Design review of the part built by this model. Coordinates are the model's own, in mm. Face numbers are marked on the shaded views. A direction names the side the tool comes from. Coordinates: 2 decimals unless noted, no trailing zeros. Order: outer loops, then holes, each group sorted by start corner. A loop starts at its lowest first (then second) coordinate and runs counter-clockwise, first axis right, second up. Notation, with made-up numbers: (-34, 72.5) -> (-11, 72.5) arc R19 ccw to (-11, 80.5) -> close; hole circle Ø2 at (-28.75, 72.5). An arc over 180 degrees is marked (long way). Use a Markdown table: item, result. Add a question column.
Q1. Add section C-C (y = 17.5). State the section outline as (x, z) points (3 decimals).
Q2. Add section B-B (z = 5). State the section outline as (x, y) points (3 decimals).
Q3. Add section A-A (x = -2.5). State the section outline as (y, z) points (3 decimals), then the cut area to 3 significant figures.
Q4. The part is to be moulded in two halves that separate along X. For the marked faces 3, 4 and 5, say which applies: pulls with the +X half, pulls with the -X half, needs draft (parallel to the pull), parting line crosses it, or undercut.
Q5. Wall thickness on probe 1 along X at (y, z) = (3.25, -34.5) (3 decimals); probe 2 along X at (y, z) = (2, 7.5) (3 decimals); probe 3 along Z at (x, y) = (34, 3.25) (3 decimals): over which ranges is each line inside the solid? List them lowest first.
Q6. Machinability: for the marked faces 1 and 2, which of the approach directions +Z, -Z, +X, -X, +Y, -Y give a long, thin tool a straight path to every point of the face, cutting with its end or side? Answer none if there is none.
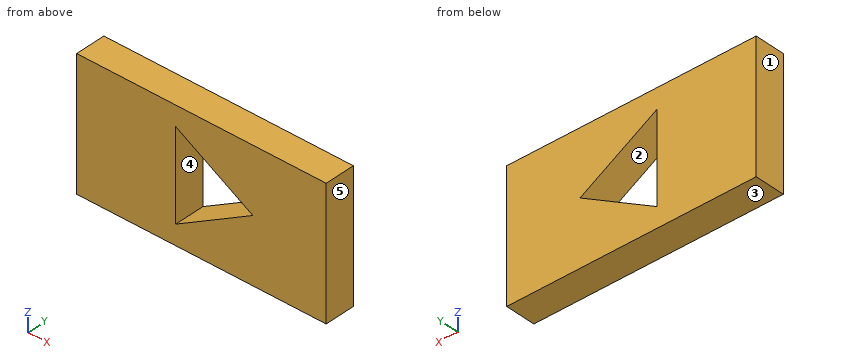
from build123d import *

# Parameters (mm, degrees)
SKETCH1_W           = 209.55
SKETCH1_H           = 107.95
BOSS_EXTRUDE1_DEPTH = 25.4


with BuildPart() as part:
    # Sketch1 → Boss-Extrude1 (new body)
    with BuildSketch(Plane(origin=(0, 0, 0), x_dir=(1, 0, 0), z_dir=(0, 1, 0))):
        Rectangle(SKETCH1_W, SKETCH1_H)
        Polygon((-21.59, 37.394976935), (-21.59, -37.394976935), (43.18, 0), align=None, mode=Mode.SUBTRACT)
    extrude(amount=BOSS_EXTRUDE1_DEPTH)


solid = part.part
Established:
| question | item | result |
|---|---|---|
| 1 | outline | (-104.775, -53.975) -> (104.775, -53.975) -> (104.775, 53.975) -> (-104.775, 53.975) -> close; hole (-21.59, -37.395) -> (43.18, 0) -> (-21.59, 37.395) -> close |
| 2 | outline | (-104.775, 0) -> (-21.59, 0) -> (-21.59, 25.4) -> (-104.775, 25.4) -> close; (34.52, 0) -> (104.775, 0) -> (104.775, 25.4) -> (34.52, 25.4) -> close |
| 3 | outline | (0, -53.975) -> (25.4, -53.975) -> (25.4, -26.373) -> (0, -26.373) -> close; (0, 26.373) -> (25.4, 26.373) -> (25.4, 53.975) -> (0, 53.975) -> close |
| 3 | area | 1,400 mm^2 |
| 4 | face 3 | needs draft |
| 4 | face 4 | undercut |
| 4 | face 5 | pulls with the +X half |
| 5 | probe 1 | -104.775 to -21.59, -16.576 to 104.775 |
| 5 | probe 2 | -104.775 to -21.59, 30.19 to 104.775 |
| 5 | probe 3 | -53.975 to -5.3, 5.3 to 53.975 |
| 6 | face 1 | +Z, -Z, -X, +Y, -Y |
| 6 | face 2 | +Y, -Y |
